Geometry: final body of the model. Coordinates: model frame, mm. A direction names the side the tool comes from. Round coordinates to 2 decimals unless told otherwise and drop trailing zeros. Order: outer loops, then holes, each group sorted by start corner. A loop starts at its lowest first (then second) coordinate and runs counter-clockwise, first axis right, second up. Notation, with made-up numbers: (80.25, 82) -> (99.25, 82) arc R29 ccw to (99.25, 109) -> close; hole circle Ø6 at (-12.75, 65). An arc over 180 degrees is marked (long way). Put each result on its own line as item: value.
```python
from build123d import *

# Parameters (mm, degrees)
F0_W         = 22.3715566099
F0_H         = 39.9701632559
F1_DEPTH     = 5.08
F2_R         = 5.7912
F3_DEPTH     = 0.762
F4_R         = 1.0769741324
F5_DEPTH     = 50.8
F6_R         = 1.8127400762
F6_R_2       = 2.5138312633
F7_DEPTH     = 0.4064
F8_SIZE      = 1.27
F9_T4_DEPTH  = 48.4998557676
F9_S5_R      = 1.0769741324
F9_T6_DEPTH  = 26
F10_SIZE     = 1.524
F11_T1_DEPTH = 27.632068852


# Not quite as in the source:
# - a fillet or chamfer that OpenCascade refuses, or shapes differently, is made with other operations: its cross-section is extruded or revolved along the edge and cut away or added


with BuildPart() as f1:
    # F0 (on Top) → F1 (new body)
    with BuildSketch(Plane.XY):
        Rectangle(F0_W, F0_H)
    extrude(amount=F1_DEPTH)

    # F2 (on Top) → F3 (cut)
    with BuildSketch(Plane.XY):
        Circle(F2_R)
    extrude(amount=F3_DEPTH, mode=Mode.SUBTRACT)

    # F4 (on Front) → F5 (join)
    with BuildSketch(Plane.XZ):
        with Locations((0, 2.4075380061)):
            Circle(F4_R)
    extrude(amount=F5_DEPTH)

    # F6 (on face) → F7 (join)
    with BuildSketch(Plane.XY.offset(5.08)):
        with Locations((-4.1463463567, 0.584599562)):
            Circle(F6_R)
        with Locations((4.7694612294, 0)):
            Circle(F6_R_2)
    extrude(amount=F7_DEPTH)

    # F8
    f8_edges = [f1.edges().sort_by_distance(p)[0] for p in [
        (0, -19.985082, 5.08),
    ]]
    chamfer(f8_edges, length=F8_SIZE)

    # F9: chamfer of 5.08 on 1 edges, made by hand


with BuildPart() as f9_tool2:
    # F9_s3 → F9_t4 (new body)
    with BuildSketch(Plane.YZ.offset(-24.2499278838)):
        Polygon((-19.985081628, 5.08), (-14.905081628, 0), (-19.985081628, 0), align=None)
    extrude(amount=F9_T4_DEPTH)

    # F9_s5 → F9_t6 (cut, symmetric)
    with BuildSketch(Plane.XZ.offset(17.4)):
        with Locations((0, 2.4075380061)):
            Circle(F9_S5_R)
    extrude(amount=F9_T6_DEPTH, both=True, mode=Mode.SUBTRACT)


with BuildPart() as f1_1:
    add(f1.part)

    # F9_t1: cut F9_tool2
    add(f9_tool2.part, mode=Mode.SUBTRACT)

    # F10
    f10_edges = [f1_1.edges().sort_by_distance(p)[0] for p in [
        (0, 19.985082, 5.08),
        (0, 19.985082, 0),
    ]]
    chamfer(f10_edges, length=F10_SIZE)

    # F11: fillet of radius 2.54 on 4 edges, made by hand

    # F11_s2 → F11_t1 (cut)
    with BuildSketch(Plane.YZ.offset(-13.816034426)):
        with BuildLine():
            ThreePointArc((17.4089791795, 5.08), (18.3809950977, 4.8866540126), (19.2050304038, 4.3360512242))
            Line((19.2050304038, 4.3360512242), (18.461081628, 5.08))
            Line((18.461081628, 5.08), (17.4089791795, 5.08))
        make_face()
        with BuildLine():
            ThreePointArc((19.2411328522, 4.2999487758), (19.7917356405, 3.4759134698), (19.985081628, 2.5038975516))
            Line((19.985081628, 2.5038975516), (19.985081628, 3.556))
            Line((19.985081628, 3.556), (19.2411328522, 4.2999487758))
        make_face()
        with BuildLine():
            ThreePointArc((19.2411328522, 0.7800512242), (19.7917356405, 1.6040865302), (19.985081628, 2.5761024484))
            Line((19.985081628, 2.5761024484), (19.985081628, 1.524))
            Line((19.985081628, 1.524), (19.2411328522, 0.7800512242))
        make_face()
        with BuildLine():
            ThreePointArc((17.4089791795, 0), (18.3809950977, 0.1933459874), (19.2050304038, 0.7439487758))
            Line((19.2050304038, 0.7439487758), (18.461081628, 0))
            Line((18.461081628, 0), (17.4089791795, 0))
        make_face()
    extrude(amount=F11_T1_DEPTH, mode=Mode.SUBTRACT)


solid = f1_1.part
```
1. Cut plane C-C on x = 4.75. Return loops of the section in (y, z) (3 decimals), and give its area (3 significant figures).
Ans:
outline: (-19.35, 4.445) -> (-14.905, 0) -> (-3.313, 0) -> (-3.313, 0.762) -> (3.313, 0.762) -> (3.313, 0) -> (17.409, 0) arc R2.54 ccw to (19.205, 0.744) -> (19.241, 0.78) arc R2.54 ccw to (19.985, 2.54) arc R2.54 ccw to (19.241, 4.3) -> (19.205, 4.336) arc R2.54 ccw to (17.409, 5.08) -> (2.514, 5.08) -> (2.514, 5.486) -> (-2.514, 5.486) -> (-2.514, 5.08) -> (-18.715, 5.08) -> close
area: 184 mm²
2. Material intervals for probe 1 along Z at (x, y) = (-3.5, 10); probe 2 along Y at (x, z) = (0, 0.4); probe 3 along Y at (x, z) = (0, 0.5), sorted ascending.
Ans:
probe 1: 0 to 5.08
probe 2: -15.31 to -5.79, 5.79 to 18.78
probe 3: -15.41 to -5.79, 5.79 to 18.92
3. Cut plane D-D on y = -24. Return loops of the section in (x, z), and give its area (3 significant figures).
Ans:
outline: circle Ø2.15 at (0, 2.41)
area: 3.64 mm²
4. Draft query along Y for faces 1 (the face through (0, 0, 5.08)), 2 (the face through (0, 0, 0.762)), 3 (the face through (-0.157, 19.779, 1.575)). Return one class per face: +Y half, -Y half, draft (parallel to the pull), parting line (faces both ways), or undercut.
Ans:
face 1: draft
face 2: undercut
face 3: +Y half
5. Set-up query: faces 4 (the face through (2.92, 1.7, 5.28)), 5 (the face through (-4, 1, 5.486)), 6 (the face through (-1.255, -5.653, 0.376)). Return all of +Z, -Z, +X, -X, +Y, -Y with unobstructed straight access to the full face (end or side cutting, diameter ignored); none if empty.
Ans:
face 4: +Z
face 5: +Z, +X, -X, +Y, -Y
face 6: -Z
6. Cut plane B-B on y = -7.5. Return loops of the section in (x, z).
Ans:
outline: (-11.19, 0) -> (11.19, 0) -> (11.19, 5.08) -> (-11.19, 5.08) -> close
7. Contact query for flat-ended pins moving along their axis: P1, Ø1, axis at x = -3, y = 11.5, coming from the +Z side; P2, Ø5, axis at x = 4, y = -36, coming from the +Z side; P3, Ø3.5, axis at x = -2.5, y = 0, coming from the -Z side. Output: stop coordinate, or through.
Ans:
P1: z = 5.08
P2: through
P3: z = 0.76
8. Cut plane A-A on x = -7.25. Return loops of the section in (y, z) (3 decimals).
Ans:
outline: (-19.35, 4.445) -> (-14.905, 0) -> (17.409, 0) arc R2.54 ccw to (19.205, 0.744) -> (19.241, 0.78) arc R2.54 ccw to (19.985, 2.54) arc R2.54 ccw to (19.241, 4.3) -> (19.205, 4.336) arc R2.54 ccw to (17.409, 5.08) -> (-18.715, 5.08) -> close
